The listing builds one solid part. Answer for the finished solid, in the listing's coordinates (mm). Face numbers are marked on the shaded views. Coordinates: 2 decimals unless noted, no trailing zeros. Order: outer loops, then holes, each group sorted by start corner. A loop starts at its lowest first (then second) coordinate and runs counter-clockwise, first axis right, second up. Notation, with made-up numbers: (45, 19.25) -> (56, 19.25) arc R15 ccw to (56, 30.25) -> close; hole circle Ø4 at (-36.75, 31). An arc over 180 degrees is marked (long way). Write item = value, one per line.
from build123d import *

# Parameters (mm, degrees)
SKETCH1_W           = 30
SKETCH1_H           = 30
BOSS_EXTRUDE1_DEPTH = 15
SKETCH3_R           = 12.5
BOSS_EXTRUDE2_DEPTH = 50
BOSS_EXTRUDE3_START = 50
SKETCH3_3_R         = 25
SKETCH3_3_R_2       = 12.5
BOSS_EXTRUDE3_DEPTH = 10
CUT_EXTRUDE1_DEPTH  = 255.656631565


with BuildPart() as part:
    # Sketch1 → Revolve1 (revolve)
    with BuildSketch(Plane(origin=(0, 0, 0), x_dir=(1, 0, 0), z_dir=(0, 1, 0)), mode=Mode.PRIVATE) as revolve1_sk:
        Polygon((-15, 175), (-15, 145), (15, 145), (15, 175), (10, 175), (0, 165), (-10, 175), align=None)
        with Locations((0, 35)):
            Rectangle(SKETCH1_W, SKETCH1_H)
    revolve(revolve1_sk.sketch.rotate(Axis((0, 0, 0), (1, 0, 0)), 180), axis=Axis((0, 0, 0), (1, 0, 0)))

    # Sketch2 → Boss-Extrude1 (add, symmetric)
    with BuildSketch(Plane(origin=(0, 0, 0), x_dir=(0, 0, -1), z_dir=(1, 0, 0))):
        with BuildLine():
            Line((25, -130.384048104), (25, -46.097722286))
            ThreePointArc((25, -46.097722286), (25.604754635, -43.714065813), (27.272727273, -41.90702026))
            ThreePointArc((27.272727273, -41.90702026), (0, -50), (-27.272727273, -41.90702026))
            ThreePointArc((-27.272727273, -41.90702026), (-25.604754635, -43.714065813), (-25, -46.097722286))
            Line((-25, -46.097722286), (-25, -130.384048104))
            ThreePointArc((-25, -130.384048104), (-28.914193805, -138.31896858), (-37.592592593, -140.042125741))
            ThreePointArc((-37.592592593, -140.042125741), (0, -145), (37.592592593, -140.042125741))
            ThreePointArc((37.592592593, -140.042125741), (28.914193805, -138.31896858), (25, -130.384048104))
        make_face()
        with BuildLine():
            ThreePointArc((-52.421798557, 1.398226049), (-50.659868815, -0.317335065), (-49.928907779, -2.665364518))
            ThreePointArc((-49.928907779, -2.665364518), (-43.301270189, 25), (-22.656180506, 44.572384779))
            ThreePointArc((-22.656180506, 44.572384779), (-25.05511418, 44.031400878), (-27.421798557, 44.699496238))
            Line((-27.421798557, 44.699496238), (-100.415897906, 86.842659147))
            ThreePointArc((-100.415897906, 86.842659147), (-105.330643713, 94.199910656), (-102.483742196, 102.57720305))
            ThreePointArc((-102.483742196, 102.57720305), (-125.573683549, 72.5), (-140.076334788, 37.464922691))
            ThreePointArc((-140.076334788, 37.464922691), (-134.244837518, 44.119057925), (-125.415897906, 43.541388957))
            Line((-125.415897906, 43.541388957), (-52.421798557, 1.398226049))
        make_face()
        with BuildLine():
            ThreePointArc((22.656180506, 44.572384779), (43.301270189, 25), (49.928907779, -2.665364518))
            ThreePointArc((49.928907779, -2.665364518), (50.659868815, -0.317335065), (52.421798557, 1.398226049))
            Line((52.421798557, 1.398226049), (125.415897906, 43.541388957))
            ThreePointArc((125.415897906, 43.541388957), (134.244837518, 44.119057925), (140.076334788, 37.464922691))
            ThreePointArc((140.076334788, 37.464922691), (125.573683549, 72.5), (102.483742196, 102.57720305))
            ThreePointArc((102.483742196, 102.57720305), (105.330643713, 94.199910656), (100.415897906, 86.842659147))
            Line((100.415897906, 86.842659147), (27.421798557, 44.699496238))
            ThreePointArc((27.421798557, 44.699496238), (25.05511418, 44.031400878), (22.656180506, 44.572384779))
        make_face()
    extrude(amount=BOSS_EXTRUDE1_DEPTH, both=True)

    # Sketch3 → Boss-Extrude2 (add)
    with BuildSketch(Plane.ZY.offset(15)):
        with Locations(Location((0, -125, 0), (0, 0, 180))):
            Circle(SKETCH3_R)
    extrude(amount=BOSS_EXTRUDE2_DEPTH)

    # Sketch3<3> → Boss-Extrude3 (add)
    # profile 1 of 2: a face of its own
    with BuildSketch(Plane.ZY.offset(15).offset(BOSS_EXTRUDE3_START)):
        with Locations((0, -125)):
            Circle(SKETCH3_3_R)
        with Locations(Location((0, -125, 0), (0, 0, 180))):
            Circle(SKETCH3_3_R_2, mode=Mode.SUBTRACT)
    # profile 2 of 2: a face of its own
    with BuildSketch(Plane.ZY.offset(15).offset(BOSS_EXTRUDE3_START)):
        with Locations(Location((0, -125, 0), (0, 0, 180))):
            Circle(SKETCH3_3_R_2)
    extrude(amount=BOSS_EXTRUDE3_DEPTH)

    # Sketch4 → Cut-Extrude1 (cut, through all)
    with BuildSketch(Plane.ZY.offset(15)):
        with BuildLine():
            Line((5, -24.364916731), (5, -19.364916731))
            ThreePointArc((5, -19.364916731), (0, -20), (-5, -19.364916731))
            Line((-5, -19.364916731), (-5, -24.364916731))
            Line((-5, -24.364916731), (5, -24.364916731))
        make_face()
    extrude(amount=-CUT_EXTRUDE1_DEPTH, mode=Mode.SUBTRACT)


solid = part.part
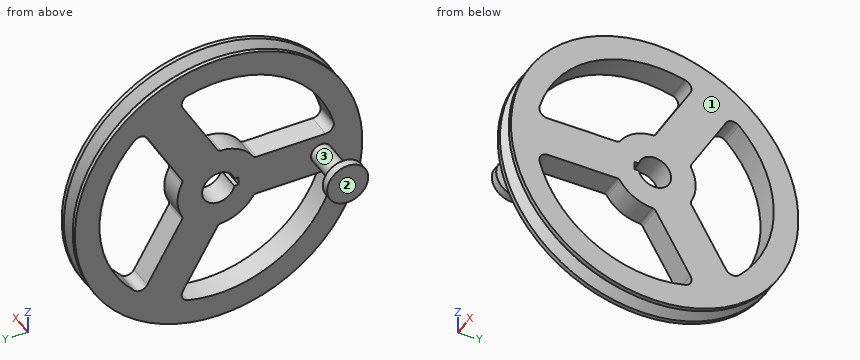
Q1. Section B-B, the plane y = -59.5 is taken. Give the number of separate pieces and of enclosed holes in the cut face, plus the area to 3 significant figures.
The answers:
separate_pieces = 3
enclosed_holes = 0
area = 3,230 mm2
Q2. Find the intervals of material crossed by line 1 along X through (y, z) = (-110.5, -4); line 2 along Z through (x, y) = (9.5, -80.5); line 3 along Y through (x, z) = (-13, 66), in increasing order.
The answers:
line_1 = -75 to -65, -15 to 15
line_2 = -154.82 to -120.6, -25 to 25, 120.6 to 154.82
line_3 = -162.08 to -129.11, 9.24 to 66.97, 129.11 to 162.08
Q3. Section A-A, the plane z = 0 is taken. Give the vertices of the cut face in (x, y), plus the area to 3 significant figures.
The answers:
outline = (-75, -150) -> (-65, -150) -> (-65, -137.5) -> (-15, -137.5) -> (-15, -175) -> (-10, -175) -> (0, -165) -> (10, -175) -> (15, -175) -> (15, -24.36) -> (-15, -24.36) -> (-15, -112.5) -> (-65, -112.5) -> (-65, -100) -> (-75, -100) -> close; (-15, 20) -> (15, 20) -> (15, 50) -> (-15, 50) -> close; (-15, 145) -> (15, 145) -> (15, 175) -> (10, 175) -> (0, 165) -> (-10, 175) -> (-15, 175) -> close
area = 7,870 mm2
Q4. Each of these flat-tipped pins is pushed along its axis until it touches: pin 1 Ø6 at (y, z) = (29.5, 90.5) entering from -X; pin 2 Ø12 at (x, z) = (-48.5, 17.5) entering from -Y; pin 3 Ø2.5 at (x, y) = (1.5, -22) entering from -Z. Where does it stop, or does it pass through?
The answers:
pin_1 = -15
pin_2 = -129.9
pin_3 = -166.31
Q5. Section C-C, the plane x = -32.5 is taken. Give the vertices of the cut face in (y, z).
The answers:
outline = circle Ø25 at (-125, 0)
Q6. The mould has two halves that part along X. Classify the marked faces 1, 2 and 3: released by +X, released by -X, zero draft, split by the parting line, or undercut.
The answers:
face_1 = released by +X
face_2 = released by -X
face_3 = undercut
